Check sheet for the drawn part. Datum: minimum x, y, z corner. Units: mm. Coordinates: 2 decimals unless noted, no trailing zeros. Write each loop counter-clockwise with the first axis right and the second up, starting at its lowest first coordinate (ties: lowest second). Pieces come first, ordered by that corner, then holes. Notation, with made-up numbers: M -28.5,-4.5 L 9.5,-4.5 A31 ccw 9.5,24.5 Z; hole C -4.5,-14.75 d1. An arc over 180 degrees is marked long. Write item = value, one per line. Start each with the question number.
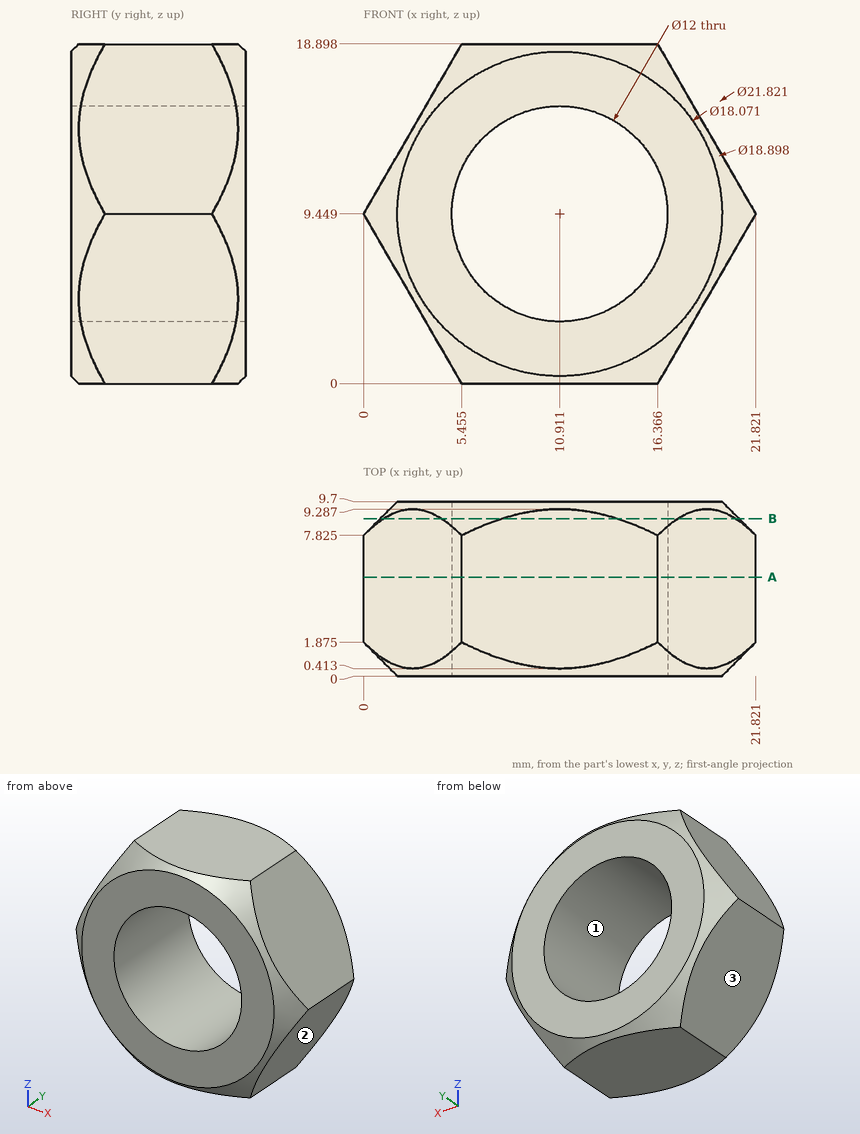
Q1. Scan lines: L1, parallel to Z at x = 10.75, y = 3; L2, parallel to X at y = 8, z = 9.25 (1 decimal); L3, parallel to Z at x = 12, y = 8.25. Record each from-to range of solid material in increasing order.
Q2. Draft check along X on the marked faces 1, 2 and 3. Enter one of: pulls with the +X half, pulls with the -X half, needs draft (parallel to the pull), parting line crosses it, or undercut.
Q3. Cross-section at B-B on y = 8.75. Enter the section's corners in (x, z) (1 decimal).
Q4. Gauge pin test, flat ends, axial feed: pin 1 (2 mm diameter, centred on y = 4, z = 14, fed in from +X); pin 2 (3 mm diameter, centred on y = 6, z = 13.5, fed in from +X); pin 3 (2 mm diameter, centred on y = 7, z = 6.5, fed in from -X) (1 decimal). Record the tip position at first contact, or that the pin passes through.
Q5. Cross-section at A-A on y = 5.5. Enter the section's corners in (x, z) (1 decimal).
Values found:
q1.L1 = 0 to 3.45, 15.45 to 18.9
q1.L2 = 0.2 to 4.9, 16.9 to 21.6
q1.L3 = 0 to 3.55, 15.35 to 18.9
q2.face_1 = undercut
q2.face_2 = pulls with the +X half
q2.face_3 = pulls with the -X half
q3.outline = M 1.1,7.5 L 4.3,1.9 A10 ccw 7.7,0 L 14.1,0 A10 ccw 17.5,1.9 L 20.7,7.5 A10 ccw 20.7,11.4 L 17.5,17 A10 ccw 14.1,18.9 L 7.7,18.9 A10 ccw 4.3,17 L 1.1,11.4 A10 ccw Z; hole C 10.9,9.4 d12
q4.pin_1 = 19.77
q4.pin_2 = 20.35
q4.pin_3 = 1.1
q5.outline = M 0,9.4 L 5.5,0 L 16.4,0 L 21.8,9.4 L 16.4,18.9 L 5.5,18.9 Z; hole C 10.9,9.4 d12
